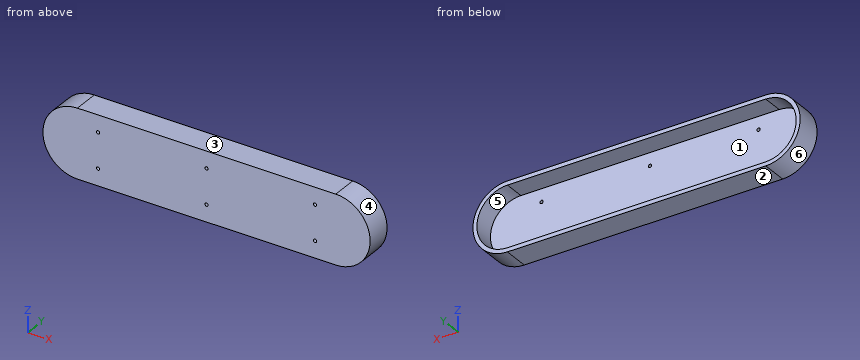
from build123d import *

# Parameters (mm, degrees)
MAINBLOCK_DEPTH     = 3.81
BOSS_EXTRUDE1_DEPTH = 19.05
SKETCH3_R           = 1.2065
CUT_EXTRUDE1_DEPTH  = 125.757705173


with BuildPart() as part:
    # Sketch1 → MainBlock (new body)
    with BuildSketch(Plane(origin=(0, 0, 0), x_dir=(1, 0, 0), z_dir=(0, 1, 0))):
        with BuildLine():
            Line((-95.25, 22.479), (95.25, 22.479))
            ThreePointArc((95.25, 22.479), (117.729, 0), (95.25, -22.479))
            Line((95.25, -22.479), (-95.25, -22.479))
            ThreePointArc((-95.25, -22.479), (-117.729, 0), (-95.25, 22.479))
        make_face()
    extrude(amount=MAINBLOCK_DEPTH)

    # Sketch2 → Boss-Extrude1 (add)
    with BuildSketch(Plane.XZ):
        with BuildLine():
            Line((-95.25, 25.4), (95.25, 25.4))
            ThreePointArc((95.25, 25.4), (120.65, 0), (95.25, -25.4))
            Line((95.25, -25.4), (-95.25, -25.4))
            ThreePointArc((-95.25, -25.4), (-120.65, 0), (-95.25, 25.4))
        make_face()
        with BuildLine():
            Line((95.25, 22.479), (-95.25, 22.479))
            ThreePointArc((-95.25, 22.479), (-117.729, 0), (-95.25, -22.479))
            Line((-95.25, -22.479), (95.25, -22.479))
            ThreePointArc((95.25, -22.479), (117.729, 0), (95.25, 22.479))
        make_face(mode=Mode.SUBTRACT)
    extrude(amount=-BOSS_EXTRUDE1_DEPTH)

    # Sketch3 → Cut-Extrude1 (cut, through all)
    with BuildSketch(Plane.XZ):
        with Locations(Location((0, 12.954, 0), (0, 0, 270))):
            Circle(SKETCH3_R)
        with Locations(Location((-80.01, 12.954, 0), (0, 0, 270))):
            Circle(SKETCH3_R)
        with Locations(Location((80.01, 12.954, 0), (0, 0, 270))):
            Circle(SKETCH3_R)
        with Locations(Location((80.01, -12.954, 0), (0, 0, 270))):
            Circle(SKETCH3_R)
        with Locations(Location((-80.01, -12.954, 0), (0, 0, 270))):
            Circle(SKETCH3_R)
        with Locations(Location((0, -12.954, 0), (0, 0, 270))):
            Circle(SKETCH3_R)
    extrude(amount=-CUT_EXTRUDE1_DEPTH, mode=Mode.SUBTRACT)


solid = part.part
Read the model definition and answer for the solid it produces. Units are mm, in the model's axes. Face numbers are marked on the shaded views. A direction names the side the tool comes from. Give positions to 0.01 mm unless a question says otherwise; leave off trailing zeros. Write each loop counter-clockwise with the first axis right and the second up, starting at its lowest first coordinate (ties: lowest second). Pieces come first, ordered by that corner, then holes. Notation, with made-up numbers: (28, -6) -> (72, -6) arc R18 ccw to (72, 8) -> close; hole circle Ø6 at (-28, 81). An arc over 180 degrees is marked (long way). Answer as a JSON object with one key per item and string values. Group by question number.
1) The mould has two halves that part along X. Classify the marked faces 3, 4, 5 and 6: +X half, -X half, draft (parallel to the pull), parting line (faces both ways), or undercut.
2) A tool of negligible diameter and unlimited length cuts with its end or side. For the marked faces 1 and 2, from which of +Z, -Z, +X, -X, +Y, -Y can it reach the whole face along a straight path? Write none if from no direction.
3) Find section A-A (y = 8.25). Write down the section's boundary in (x, z), and give its area (3 significant figures).
4) Each of these flat-tipped pins is pushed along its axis until it touches: P1, Ø1.5, axis at y = 13.5, z = 7, coming from the +X side; P2, Ø4, axis at x = 0, z = -12.954, coming from the +Y side; P3, Ø1.4, axis at x = 0, z = 12.954, coming from the -Y side; P4, Ø5, axis at y = 13, z = -19, coming from the -X side. Where does it stop, or does it pass through?
5) Consider L1, parallel to Z at x = 80.01, y = 2.8; L2, parallel to Z at x = 61, y = 12; L3, parallel to Y at x = -51.5, z = -2. Determine where each line is inside the solid, lowest interval first. Write a range as from..to.
6) Find section C-C (x = -5). Write down the section's boundary in (y, z), and give its area (3 significant figures).
7) Find section B-B (z = 0). Write down the section's boundary in (x, y).
Values follow:
{
 "1": {"face 3": "draft", "face 4": "+X half", "face 5": "undercut", "face 6": "-X half"},
 "2": {"face 1": "+Y", "face 2": "-Z, +X, -X, +Y, -Y"},
 "3": {"outline": "(-95.25, -25.4) -> (95.25, -25.4) arc R25.4 ccw to (95.25, 25.4) -> (-95.25, 25.4) arc R25.4 ccw to start; hole (-95.25, -22.48) -> (95.25, -22.48) arc R22.48 ccw to (95.25, 22.48) -> (-95.25, 22.48) arc R22.48 ccw to start", "area": "1,550 mm2"},
 "4": {"P1": "stops at x = 119.87", "P2": "stops at y = 3.81", "P3": "passes through", "P4": "stops at x = -114.56"},
 "5": {"L1": "z = -25.4..-14.16, -11.75..11.75, 14.16..25.4", "L2": "z = -25.4..-22.48, 22.48..25.4", "L3": "y = 0..3.81"},
 "6": {"outline": "(0, -25.4) -> (19.05, -25.4) -> (19.05, -22.48) -> (3.81, -22.48) -> (3.81, 22.48) -> (19.05, 22.48) -> (19.05, 25.4) -> (0, 25.4) -> close", "area": "283 mm2"},
 "7": {"outline": "(-120.65, 0) -> (120.65, 0) -> (120.65, 19.05) -> (117.73, 19.05) -> (117.73, 3.81) -> (-117.73, 3.81) -> (-117.73, 19.05) -> (-120.65, 19.05) -> close"}
}
